from build123d import *

# Parameters (mm, degrees)
BOSS_EXTRUDE1_DEPTH      = 24
BOSS_EXTRUDE1_DEPTH_BACK = 57
SKETCH1_R                = 18.5
SKETCH2_R                = 1.5
CUT_EXTRUDE1_DEPTH       = 5
SKETCH3_R                = 6
SKETCH3_R_2              = 3
BOSS_EXTRUDE2_DEPTH      = 6
SKETCH3_2_R              = 3
BOSS_EXTRUDE3_DEPTH      = 21


with BuildPart() as part:
    # Sketch1 → Boss-Extrude1 (new, two sides: drawn at the far end of the back side and taken through both)
    with BuildSketch(Plane.XY.offset(-BOSS_EXTRUDE1_DEPTH_BACK)):
        Circle(SKETCH1_R)
    extrude(amount=BOSS_EXTRUDE1_DEPTH + BOSS_EXTRUDE1_DEPTH_BACK)

    # Sketch2 → Cut-Extrude1 (cut)
    with BuildSketch(Plane.XY.offset(24)):
        with Locations((15.5, 0)):
            Circle(SKETCH2_R)
        with Locations((7.75, -13.423393759)):
            Circle(SKETCH2_R)
        with Locations((-7.75, -13.423393759)):
            Circle(SKETCH2_R)
        with Locations((-15.5, 0)):
            Circle(SKETCH2_R)
        with Locations((-7.75, 13.423393759)):
            Circle(SKETCH2_R)
        with Locations((7.75, 13.423393759)):
            Circle(SKETCH2_R)
    extrude(amount=-CUT_EXTRUDE1_DEPTH, mode=Mode.SUBTRACT)

    # Sketch3 → Boss-Extrude2 (add)
    with BuildSketch(Plane.XY.offset(24)):
        with Locations((0, 7)):
            Circle(SKETCH3_R)
        with Locations((0, 7)):
            Circle(SKETCH3_R_2, mode=Mode.SUBTRACT)
    extrude(amount=BOSS_EXTRUDE2_DEPTH)

    # Sketch3_2 → Boss-Extrude3 (add)
    with BuildSketch(Plane.XY.offset(24)):
        with Locations(Location((0, 7, 0), (0, 0, 180))):
            Circle(SKETCH3_2_R)
    extrude(amount=BOSS_EXTRUDE3_DEPTH)


solid = part.part
Geometry: final body of the model. Coordinates: model frame, mm. A direction names the side the tool comes from. Give positions to 0.01 mm unless a question says otherwise; leave off trailing zeros. Write each loop counter-clockwise with the first axis right and the second up, starting at its lowest first coordinate (ties: lowest second). Pieces come first, ordered by that corner, then holes.
(1) First-contact query: P1, Ø1.8, axis at x = -7.75, y = -13.42, coming from the +Z side; P2, Ø4, axis at x = -3.5, z = -33.5, coming from the -Y side; P3, Ø10, axis at x = -10.5, z = -5.5, coming from the +Y side. Flat tips, straight axial feed; report the tip coordinate or a pass-through.
(2) Cut plane B-B, the plane y = 7. Return loops of the section in (x, z), then the cut area to 3 significant figures.
(3) Cut plane C-C, the plane z = 4. Return loops of the section in (x, y), then the cut area to 3 significant figures.
(4) Cut plane D-D, the plane x = 15.5. Return loops of the section in (y, z).
(5) Access query for faces 5 (the flat face through (-8, -13, 19)), 6 (the cylindrical face through (-4.01, -18.06, -17.07)). Directions: +Z, -Z, +X, -X, +Y, -Y. A direction counts if a zero-diameter tool reaches every point of the face in a straight line with its end or side. Return the directions, or none.
(6) Mould query, pull axis X, two halves, no side actions, for faces 1 (the flat face through (-16, 0, 19)), 2 (the cylindrical face through (-0.78, 12.95, 26.96)), 3 (the flat face through (0, 0, -57)), 4 (the flat face through (15, 0, 19)). Classes: released by +X, released by -X, zero draft, split by the parting line, or undercut.
(7) Ray query, line 1 (Y direction, x = -8, z = 22); line 2 (Y direction, x = 7.75, z = 23); line 3 (Z direction, x = 9, y = 0). Return the intervals inside material, ascending.
(8) Cut plane A-A, the plane x = -2. Return loops of the section in (y, z).
Values follow:
1. P1: stops at z = 19
1. P2: stops at y = -18.44
1. P3: stops at y = 17.66
2. outline: (-17.12, -57) - (17.12, -57) - (17.12, 24) - (6, 24) - (6, 30) - (3, 30) - (3, 45) - (-3, 45) - (-3, 30) - (-6, 30) - (-6, 24) - (-17.12, 24) - close
2. area: 2,940 mm2
3. outline: circle Ø37 at (0, 0)
3. area: 1,080 mm2
4. outline: (-10.1, -57) - (10.1, -57) - (10.1, 24) - (1.5, 24) - (1.5, 19) - (-1.5, 19) - (-1.5, 24) - (-10.1, 24) - close
5. face 5: +Z
5. face 6: +Z, -Z
6. face 1: undercut
6. face 2: split by the parting line
6. face 3: zero draft
6. face 4: undercut
7. line 1: y = -16.68 to -14.9, -11.94 to 11.94, 14.9 to 16.68
7. line 2: y = -16.8 to -14.92, -11.92 to 11.92, 14.92 to 16.8
7. line 3: z = -57 to 24
8. outline: (-18.39, -57) - (18.39, -57) - (18.39, 24) - (12.66, 24) - (12.66, 30) - (9.24, 30) - (9.24, 45) - (4.76, 45) - (4.76, 30) - (1.34, 30) - (1.34, 24) - (-18.39, 24) - close
